```python
from build123d import *

# Parameters (mm, degrees)
SKETCH119_W             = 47
SKETCH119_H             = 52
SKETCH119_W_2           = 37
SKETCH119_H_2           = 42
PAD060_DEPTH            = 135
SKETCH120_W             = 42.5
SKETCH120_H             = 47
POCKET051_DEPTH         = 7
SKETCH118_W             = 23
SKETCH118_H             = 2.25
POCKET052_DEPTH         = 15
BODY033_PLACEMENT_ANGLE = 180


with BuildPart() as part:
    # Sketch119 → Pad060 (new body)
    with BuildSketch(Plane.XY):
        with Locations((0, -26)):
            Rectangle(SKETCH119_W, SKETCH119_H)
        with Locations((0, -26)):
            Rectangle(SKETCH119_W_2, SKETCH119_H_2, mode=Mode.SUBTRACT)
    extrude(amount=PAD060_DEPTH)

    # Sketch120 (on Face10 of Pad060) → Pocket051 (cut)
    with BuildSketch(Plane.XY.offset(135)):
        with Locations((0, -25.75)):
            Rectangle(SKETCH120_W, SKETCH120_H)
    extrude(amount=-POCKET051_DEPTH, mode=Mode.SUBTRACT)

    # Sketch118 (on Face15 of Pocket051) → Pocket052 (cut)
    with BuildSketch(Plane.XY.offset(128)):
        with Locations((0, -48.125)):
            Rectangle(SKETCH118_W, SKETCH118_H)
    extrude(amount=-POCKET052_DEPTH, mode=Mode.SUBTRACT)


with BuildPart() as part_1:
    # Body033 placement: moved
    add(part.part.rotate(Axis((0, 0, 0), (0, 0, 1)), BODY033_PLACEMENT_ANGLE))


solid = part_1.part
```
The model under review builds one solid part; all positions refer to its coordinate system, in mm. A direction names the side the tool comes from. Round coordinates to 2 decimals unless told otherwise and drop trailing zeros. Loops run counter-clockwise (first coordinate to the right, second up) from the corner with the lowest first, then second, coordinate; pieces in that order, holes last. Notation, with made-up numbers: M 76.5,-2.5 L 88.5,-2.5 A29 ccw 88.5,31.5 Z; hole C 76.25,72.25 d10. An arc over 180 degrees is marked long. Answer as a JSON object with one key per item and string values.
(1) Take a section at B-B on z = 53. Give the boundary of the cut face in (x, y).
Resolved:
{"outline": "M -23.5,0 L 23.5,0 L 23.5,52 L -23.5,52 Z; hole M -18.5,5 L 18.5,5 L 18.5,47 L -18.5,47 Z"}
(2) Take a section at D-D on z = 119. Give the boundary of the cut face in (x, y), and give its area (3 significant figures).
Resolved:
{"outline": "M -23.5,0 L 23.5,0 L 23.5,52 L -23.5,52 Z; hole M -18.5,5 L 18.5,5 L 18.5,47 L 11.5,47 L 11.5,49.25 L -11.5,49.25 L -11.5,47 L -18.5,47 Z", "area": "838 mm²"}
(3) Take a section at C-C on y = 42.5. Give the boundary of the cut face in (x, z).
Resolved:
{"outline": "M -23.5,0 L -18.5,0 L -18.5,128 L -21.25,128 L -21.25,135 L -23.5,135 Z; M 18.5,0 L 23.5,0 L 23.5,135 L 21.25,135 L 21.25,128 L 18.5,128 Z"}
(4) Draft analysis for pull direction X (two halves, no side actions). For faces 4 (the flat face through (-21, 26, 0)), 5 (the flat face through (23.5, 26, 67)), 6 (the flat face through (-21.25, 26, 132)), state which applies: released by +X, released by -X, zero draft, split by the parting line, or undercut.
Resolved:
{"face 4": "zero draft", "face 5": "released by +X", "face 6": "undercut"}
(5) To check wall thickness, follow line 1 along X through (y, z) = (33, 112); line 2 along Y through (x, z) = (-14, 42.5); line 3 along Z through (x, y) = (20.5, 34). State the ranges of each line that lie inside material, in increasing order.
Resolved:
{"line 1": "-23.5 to -18.5, 18.5 to 23.5", "line 2": "0 to 5, 47 to 52", "line 3": "0 to 128"}
(6) Tool access review of faces 1 (the flat face through (18.5, 26, 63)), 2 (the flat face through (-23.5, 26, 67)), 3 (the flat face through (0, 2.25, 132)): name each direction out of +Z, -Z, +X, -X, +Y, -Y from which nothing blocks a thin tool from reaching the whole face with its end or side.
Resolved:
{"face 1": "+Z, -Z", "face 2": "+Z, -Z, -X, +Y, -Y", "face 3": "+Z"}
(7) Clearance check with a flat-ended pin moving along its axis: P1, Ø1.1, axis at x = 2, y = 48, coming from the +Z side. State where the tip first meets the part, or that it passes through.
Resolved:
{"P1": "z = 113"}
(8) Take a section at A-A on x = -6. Give the boundary of the cut face in (y, z), and give its area (3 significant figures).
Resolved:
{"outline": "M 0,0 L 5,0 L 5,128 L 2.25,128 L 2.25,135 L 0,135 Z; M 47,0 L 52,0 L 52,135 L 49.25,135 L 49.25,113 L 47,113 Z", "area": "1,280 mm²"}
